Design review of the part built by this model. Coordinates are the model's own, in mm. A direction names the side the tool comes from. Coordinates: 2 decimals unless noted, no trailing zeros. Loops run counter-clockwise (first coordinate to the right, second up) from the corner with the lowest first, then second, coordinate; pieces in that order, holes last. Notation, with made-up numbers: (77.25, 64) - (102.25, 64) arc R26 ccw to (102.25, 99) - close; hole circle Ø3 at (80, 81). An arc over 180 degrees is marked (long way). Answer in a Markdown table with one row per item. Add a question column.
(1) For faces 5 (the face through (9, -6.35, 1)), 6 (the face through (1.4, -6.55, 4.8)), 7 (the face through (-2, -7.75, 2)), 8 (the face through (-9, 6.35, 1)), list the 3-axis set-ups (+Z, -Z, +X, -X, +Y, -Y) from which the entire face can be reached by the end or side of a thin tool; tool diameter is ignored.
(2) We need section D-D, the plane z = 6.35. Write out the cut boundary in (x, y), plus the area to 3 significant figures.
(3) We need section A-A, the plane x = 0. Write out the cut boundary in (y, z).
(4) We need section C-C, the plane y = 5.25. Write out the cut boundary in (x, z).
(5) We need section B-B, the plane y = 0. Write out the cut boundary in (x, z), plus the area to 3 significant figures.
(6) The part is to be moulded in two halves that separate along X. For faces 1 (the face through (19.05, -0.14, 0.64)), 2 (the face through (-19.05, 0.14, 0.64)), 3 (the face through (3.35, 0, 6)), 4 (the face through (10, 0, 1.3)), say which applies: released by +X, released by -X, zero draft, split by the parting line, or undercut.
(7) Clearance check with flat-ended pins moving along their axes: pin 1 (1 mm diameter, centred on x = -8, z = 1, fed in from +Y); pin 2 (4 mm diameter, centred on x = -12.5, y = -2, fed in from +Z); pin 3 (6 mm diameter, centred on y = 3.5, z = 4, fed in from +X). State where each tip first meets the part, or that it passes through.
(8) To check wall thickness, follow L1, parallel to Z at x = 0, y = -9.05; L2, parallel to X at y = -0.5, z = 3.5; L3, parallel to Y at x = 1, z = 12.25. State the ranges of each line that lie inside material, in increasing order. Write a range as [from, to].
from build123d import *

# Parameters (mm, degrees)
PAD_DEPTH       = 1.3
SKETCH001_W     = 9.1
SKETCH001_H     = 15.5
PAD001_DEPTH    = 12.7
SKETCH002_W     = 6.7
SKETCH002_H     = 13.1
POCKET_DEPTH    = 12.701
SKETCH003_R     = 2.15
POCKET001_DEPTH = 98.797458
SKETCH004_R     = 4.5
PAD002_DEPTH    = 2.7
SKETCH005_R     = 1.6
POCKET002_DEPTH = 3.9
FILLET_R        = 0.5


with BuildPart() as part:
    # Sketch → Pad (new body)
    with BuildSketch(Plane.XY):
        with BuildLine():
            ThreePointArc((-12.7, 6.35), (-19.05, 0), (-12.7, -6.35))
            Line((-12.7, -6.35), (12.7, -6.35))
            ThreePointArc((12.7, -6.35), (19.05, 0), (12.7, 6.35))
            Line((-12.7, 6.35), (12.7, 6.35))
        make_face()
    extrude(amount=PAD_DEPTH)

    # Sketch001 → Pad001 (join)
    with BuildSketch(Plane.XY):
        Rectangle(SKETCH001_W, SKETCH001_H)
    extrude(amount=PAD001_DEPTH)

    # Sketch002 → Pocket (cut, through all)
    with BuildSketch(Plane.XY):
        Rectangle(SKETCH002_W, SKETCH002_H)
    extrude(amount=POCKET_DEPTH, mode=Mode.SUBTRACT)

    # Sketch003 → Pocket001 (cut, through all)
    with BuildSketch(Plane.XY):
        with Locations((-12.7, 0)):
            Circle(SKETCH003_R)
    pocket001 = extrude(amount=POCKET001_DEPTH, mode=Mode.SUBTRACT)

    # Mirrored: Pocket001 across Sketch003 V_Axis
    add(pocket001.mirror(Plane(origin=(0, 0, 0), x_dir=(0, 0, 1), z_dir=(1, 0, 0))), mode=Mode.SUBTRACT)

    # Sketch004 (on Face11 of Mirrored) → Pad002 (join)
    with BuildSketch(Plane.XZ.offset(7.75)):
        with Locations((0, 6.35)):
            Circle(SKETCH004_R)
    extrude(amount=PAD002_DEPTH)

    # Sketch005 (on Face25 of Pad002) → Pocket002 (cut)
    with BuildSketch(Plane.XZ.offset(10.45)):
        with Locations((0, 6.35)):
            Circle(SKETCH005_R)
    extrude(amount=-POCKET002_DEPTH, mode=Mode.SUBTRACT)

    # Fillet
    fillet_edges = [part.edges().sort_by_distance(p)[0] for p in [
        (-4.5, -10.45, 6.35),
    ]]
    fillet(fillet_edges, radius=FILLET_R)


solid = part.part
Responses:
| question | item | result |
|---|---|---|
| 1 | face 5 | +Z, -Z, +X, -Y |
| 1 | face 6 | +Z, -Z |
| 1 | face 7 | -Y |
| 1 | face 8 | +Z, -Z, -X, +Y |
| 2 | outline | (-4.55, -7.75) - (-4.5, -7.75) - (-4.5, -9.95) arc R0.5 ccw to (-4, -10.45) - (-1.6, -10.45) - (-1.6, -6.55) - (-3.35, -6.55) - (-3.35, 6.55) - (3.35, 6.55) - (3.35, -6.55) - (1.6, -6.55) - (1.6, -10.45) - (4, -10.45) arc R0.5 ccw to (4.5, -9.95) - (4.5, -7.75) - (4.55, -7.75) - (4.55, 7.75) - (-4.55, 7.75) - close |
| 2 | area | 65.0 mm2 |
| 3 | outline | (-10.45, 2.35) arc R0.5 ccw to (-9.95, 1.85) - (-7.75, 1.85) - (-7.75, 0) - (-6.55, 0) - (-6.55, 4.75) - (-10.45, 4.75) - close; (-10.45, 7.95) - (-6.55, 7.95) - (-6.55, 12.7) - (-7.75, 12.7) - (-7.75, 10.85) - (-9.95, 10.85) arc R0.5 ccw to (-10.45, 10.35) - close; (6.55, 0) - (7.75, 0) - (7.75, 12.7) - (6.55, 12.7) - close |
| 4 | outline | (-16.27, 0) - (-3.35, 0) - (-3.35, 12.7) - (-4.55, 12.7) - (-4.55, 1.3) - (-16.27, 1.3) - close; (3.35, 0) - (16.27, 0) - (16.27, 1.3) - (4.55, 1.3) - (4.55, 12.7) - (3.35, 12.7) - close |
| 5 | outline | (-19.05, 0) - (-14.85, 0) - (-14.85, 1.3) - (-19.05, 1.3) - close; (-10.55, 0) - (-3.35, 0) - (-3.35, 12.7) - (-4.55, 12.7) - (-4.55, 1.3) - (-10.55, 1.3) - close; (3.35, 0) - (10.55, 0) - (10.55, 1.3) - (4.55, 1.3) - (4.55, 12.7) - (3.35, 12.7) - close; (14.85, 0) - (19.05, 0) - (19.05, 1.3) - (14.85, 1.3) - close |
| 5 | area | 57.0 mm2 |
| 6 | face 1 | released by +X |
| 6 | face 2 | released by -X |
| 6 | face 3 | undercut |
| 6 | face 4 | zero draft |
| 7 | pin 1 | stops at y = 6.35 |
| 7 | pin 2 | stops at z = 1.3 |
| 7 | pin 3 | stops at x = 18.66 |
| 8 | L1 | z = [1.85, 4.75], [7.95, 10.85] |
| 8 | L2 | x = [-4.55, -3.35], [3.35, 4.55] |
| 8 | L3 | y = [-7.75, -6.55], [6.55, 7.75] |
